from build123d import *

# Parameters (mm, degrees)
BASE_GEO_DEPTH                  = 15.875
SKETCH2_R                       = 3.5000057
BOLT_HOLE_DEPTH                 = 40.033000837
SKETCH3_R                       = 5.7500012
NUT_AND_BOLT_HEAD_CUTOUTS_DEPTH = 33.953001
SKETCH5_W                       = 177.8
SKETCH5_H                       = 19.05
BOSS_EXTRUDE1_DEPTH             = 31.75
CUT_EXTRUDE1_DEPTH              = 32.75
CHAMFER1_SIZE                   = 5.08


with BuildPart() as part:
    # Sketch1 → base geo (new body, symmetric)
    with BuildSketch(Plane.XY):
        with BuildLine():
            ThreePointArc((-78.359, 0), (0, -78.359), (78.359, 0))
            Line((78.359, 0), (119.634, 0))
            Line((119.634, 0), (119.634, -39.033000837))
            Line((119.634, -39.033000837), (94.234, -39.033000837))
            Line((94.234, -39.033000837), (39.033000837, -94.234))
            Line((39.033000837, -94.234), (39.033000837, -119.634))
            Line((39.033000837, -119.634), (-39.033000837, -119.634))
            Line((-39.033000837, -119.634), (-39.033000837, -94.234))
            Line((-39.033000837, -94.234), (-94.234, -39.033000837))
            Line((-94.234, -39.033000837), (-119.634, -39.033000837))
            Line((-119.634, -39.033000837), (-119.634, 0))
            Line((-119.634, 0), (-78.359, 0))
        make_face()
    extrude(amount=BASE_GEO_DEPTH, both=True)

    # Sketch2 → bolt hole (cut, through all)
    with BuildSketch(Plane.XZ.offset(39.033000837)):
        with Locations((-106.934, 0)):
            Circle(SKETCH2_R)
    bolt_hole = extrude(amount=-BOLT_HOLE_DEPTH, mode=Mode.SUBTRACT)

    # bolt hole mirrored: bolt hole across plane
    add(bolt_hole.mirror(Plane(origin=(0, 0, 0), x_dir=(0, 0, 1), z_dir=(1, 0, 0))), mode=Mode.SUBTRACT)

    # Sketch3 → nut and bolt head cutouts (cut)
    with BuildSketch(Plane.XZ.offset(39.033000837)):
        with Locations((-106.934, 0)):
            Circle(SKETCH3_R)
        Polygon((112.1840022, -3.031090183), (112.1840022, 3.031090183), (106.934, 6.062180367), (101.6839978, 3.031090183), (101.6839978, -3.031090183), (106.934, -6.062180367), align=None)
    extrude(amount=-NUT_AND_BOLT_HEAD_CUTOUTS_DEPTH, mode=Mode.SUBTRACT)

    # Sketch5 → Boss-Extrude1 (add)
    with BuildSketch(Plane(origin=(0, 0, -15.875), x_dir=(-1, 0, 0), z_dir=(0, 0, -1))):
        with Locations((0, -129.159)):
            Rectangle(SKETCH5_W, SKETCH5_H)
    extrude(amount=-BOSS_EXTRUDE1_DEPTH)

    # Sketch6 → Cut-Extrude1 (cut, through all)
    with BuildSketch(Plane(origin=(0, 0, -15.875), x_dir=(-1, 0, 0), z_dir=(0, 0, -1))):
        with BuildLine():
            Line((12.7, -120.65), (-12.7, -120.65))
            ThreePointArc((-12.7, -120.65), (-17.190128061, -118.790128061), (-19.05, -114.3))
            Line((-19.05, -114.3), (-19.05, -95.25))
            ThreePointArc((-19.05, -95.25), (-17.190128061, -90.759871939), (-12.7, -88.9))
            Line((-12.7, -88.9), (12.7, -88.9))
            ThreePointArc((12.7, -88.9), (17.190128061, -90.759871939), (19.05, -95.25))
            Line((19.05, -95.25), (19.05, -114.3))
            ThreePointArc((19.05, -114.3), (17.190128061, -118.790128061), (12.7, -120.65))
        make_face()
    extrude(amount=-CUT_EXTRUDE1_DEPTH, mode=Mode.SUBTRACT)

    # Chamfer1
    chamfer1_edges = [part.edges().sort_by_distance(p)[0] for p in [
        (39.033000837, -119.634, 0),
        (-39.033000837, -119.634, 0),
    ]]
    chamfer(chamfer1_edges, length=CHAMFER1_SIZE)


solid = part.part
Can you work these out from the model? Positions are in its coordinate system, mm. A direction names the side the tool comes from. Give positions to 0.01 mm unless a question says otherwise; leave off trailing zeros. Order: outer loops, then holes, each group sorted by start corner. A loop starts at its lowest first (then second) coordinate and runs counter-clockwise, first axis right, second up. Notation, with made-up numbers: M -38.5,-38.75 L 19.5,-38.75 A27 ccw 19.5,-22.75 Z; hole C 30.5,70 d7. An arc over 180 degrees is marked long. One line per item, written item: value.
Item 1: For pin 1 (7.5 mm diameter, centred on x = -105.5, z = -2, fed in from -Y); pin 2 (6 mm diameter, centred on y = -107, z = 3, fed in from +X); pin 3 (9.5 mm diameter, centred on x = -62.5, z = -6, fed in from +Y), each with a flat end and sliding along its axis, tell me the tip position at first contact or that it passes through.
Verdict:
pin 1: y = -39.03
pin 2: x = 39.03
pin 3: y = -40.22
Item 2: If we section it at C-C on x = 41.5: Write out the boundary of the cut face in (y, z) (3 decimals).
Verdict:
outline: M -138.684,-15.875 L -117.021,-15.875 L -117.021,15.875 L -138.684,15.875 Z; M -91.767,-15.875 L -66.467,-15.875 L -66.467,15.875 L -91.767,15.875 Z
Item 3: If we section it at A-A on y = -12: Write out the boundary of the cut face in (x, z) (3 decimals).
Verdict:
outline: M -119.634,-15.875 L -77.435,-15.875 L -77.435,15.875 L -119.634,15.875 Z; M 77.435,-15.875 L 119.634,-15.875 L 119.634,15.875 L 77.435,15.875 Z; hole C -106.934,0 d11.5; hole M 101.684,-3.031 L 106.934,-6.062 L 112.184,-3.031 L 112.184,3.031 L 106.934,6.062 L 101.684,3.031 Z
Item 4: If we mould it in two halves opening along Z, with no side actions, what happens to faces 1 (the face through (-17.14, -90.71, -0.22)), 2 (the face through (1, -79, -15.875)), 3 (the face through (109.52, -22.29, -4.57))? For each: pulls with the +Z half, pulls with the -Z half, needs draft (parallel to the pull), parting line crosses it, or undercut.
Verdict:
face 1: needs draft
face 2: pulls with the -Z half
face 3: undercut
Item 5: If we section it at B-B on z = 0: State how many separate pieces and enclosed holes the cut face has, and give its area (3 significant figures).
Verdict:
separate pieces: 3
enclosed holes: 1
area: 10,500 mm2
Item 6: If we section it at D-D on z = 10.5: Write out the boundary of the cut face in (x, y), and give its area (3 significant figures).
Verdict:
outline: M -119.63,-39.03 L -94.23,-39.03 L -39.03,-94.23 L -39.03,-114.55 L -44.11,-119.63 L -88.9,-119.63 L -88.9,-138.68 L 88.9,-138.68 L 88.9,-119.63 L 44.11,-119.63 L 39.03,-114.55 L 39.03,-94.23 L 94.23,-39.03 L 119.63,-39.03 L 119.63,0 L 78.36,0 A78.36 cw -78.36,0 L -119.63,0 Z; hole M -19.05,-114.3 A6.35 ccw -12.7,-120.65 L 12.7,-120.65 A6.35 ccw 19.05,-114.3 L 19.05,-95.25 A6.35 ccw 12.7,-88.9 L -12.7,-88.9 A6.35 ccw -19.05,-95.25 Z
area: 11,300 mm2
Item 7: For faces 4 (the face through (39.033, -104, 0)), 5 (the face through (-39.033, -105, 0)), 6 (the face through (88.9, -129, 0)), which set-ups out of +Z, -Z, +X, -X, +Y, -Y let a thin tool reach every point of the face, with its end or its side?
Verdict:
face 4: +Z, -Z, +X
face 5: +Z, -Z, -X
face 6: +Z, -Z, +X, -Y
Item 8: Please list where these lines run through material, in increasing order: line 1 (X direction, y = -96, z = 7); line 2 (Y direction, x = 14.5, z = -6.5); line 3 (Y direction, x = -81, z = -1.5).
Verdict:
line 1: -39.03 to -19.05, 19.05 to 39.03
line 2: -138.68 to -120.39, -89.16 to -77.01
line 3: -138.68 to -119.63, -52.27 to 0
